```python
from build123d import *

# Parameters (mm, degrees)
SKETCH1_W           = 30
SKETCH1_H           = 5.5
BOSS_EXTRUDE2_DEPTH = 5.5
FILLET1_R           = 3
FILLET2_R           = 3


with BuildPart() as part:
    # Sketch1 → Boss-Extrude2 (new body)
    with BuildSketch(Plane.XY):
        Polygon((78.5, 0), (137, 0), (142.5, 0), (142.5, 10), (137, 10), (137, 20), (129, 20), (129, 18.8), (126, 18.8), (126, 20), (123, 20), (123, 23), (126, 23), (126, 24.2), (129, 24.2), (129, 23), (137, 23), (137, 68), (142.5, 68), (142.5, 78), (137, 78), (0, 78), (-5.5, 78), (-5.5, 68), (0, 68), (0, 23), (8, 23), (8, 24.2), (11, 24.2), (11, 23), (14, 23), (14, 20), (11, 20), (11, 18.8), (8, 18.8), (8, 20), (0, 20), (0, 10), (-5.5, 10), (-5.5, 0), (0, 0), (58.5, 0), (58.5, -5), (78.5, -5), align=None)
        with Locations((68.5, 72.75)):
            Rectangle(SKETCH1_W, SKETCH1_H, mode=Mode.SUBTRACT)
    extrude(amount=BOSS_EXTRUDE2_DEPTH)

    # Fillet1
    fillet1_edges = [part.edges().sort_by_distance(p)[0] for p in [
        (78.5, -5, 2.75),
    ]]
    fillet(fillet1_edges, radius=FILLET1_R)

    # Fillet2
    fillet2_edges = [part.edges().sort_by_distance(p)[0] for p in [
        (58.5, -5, 2.75),
    ]]
    fillet(fillet2_edges, radius=FILLET2_R)


solid = part.part
```
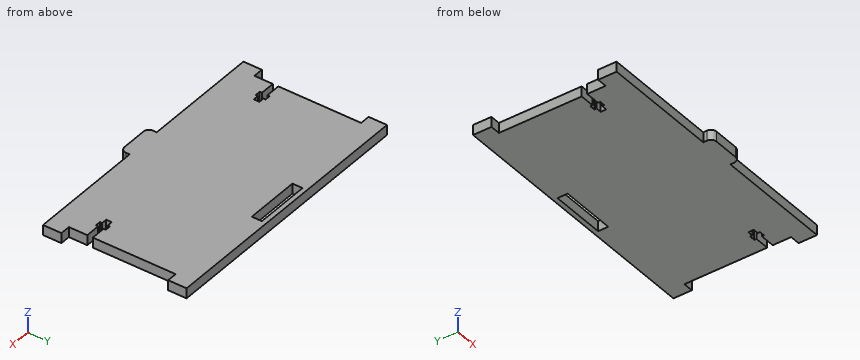
Geometry check sheet. Reference: the model listing, model coordinates, mm. Coordinates: 2 decimals unless noted, no trailing zeros. Write each loop counter-clockwise with the first axis right and the second up, starting at its lowest first coordinate (ties: lowest second). Pieces come first, ordered by that corner, then holes. Notation, with made-up numbers: M 82.25,-15 L 99.25,-15 A26 cw 99.25,8 Z; hole C 15.25,68.5 d3. An arc over 180 degrees is marked long. One line per item, written item: value. Start each with the question number.
(1) Depth check by flat-ended pin: pin 1 (1 mm diameter, centred on y = 24, z = 3, fed in from -X); pin 2 (2.5 mm diameter, centred on y = 21, z = 3, fed in from +X); pin 3 (0.9 mm diameter, centred on x = 9.5, z = 1.5, fed in from -Y). Enter the tip coordinate at first touch or a pass-through.
(2) Scan lines: line 1 along Y through (x, z) = (132, 2.7); line 2 along Y through (x, z) = (57, 0.75); line 3 along Y through (x, z) = (35.5, 3.75). Record each from-to range of solid material in increasing order. Write a range as [from, to].
(3) Sectioned sample at B-B, the plane y = 56. Enter the section's corners in (x, z).
(4) Sectioned sample at D-D, the plane x = 23. Enter the section's corners in (y, z).
(5) Sectioned sample at C-C, the plane x = 60. Enter the section's corners in (y, z).
(6) Sectioned sample at A-A, the plane x = 132.5. Enter the section's corners in (y, z).
Filled sheet:
1. pin 1: x = 0
1. pin 2: x = 137
1. pin 3: y = 0
2. line 1: [0, 20], [23, 78]
2. line 2: [0, 70], [75.5, 78]
2. line 3: [0, 78]
3. outline: M 0,0 L 137,0 L 137,5.5 L 0,5.5 Z
4. outline: M 0,0 L 78,0 L 78,5.5 L 0,5.5 Z
5. outline: M -4.6,0 L 70,0 L 70,5.5 L -4.6,5.5 Z; M 75.5,0 L 78,0 L 78,5.5 L 75.5,5.5 Z
6. outline: M 0,0 L 20,0 L 20,5.5 L 0,5.5 Z; M 23,0 L 78,0 L 78,5.5 L 23,5.5 Z
